Check sheet for the modelled part. Datum: model origin and axes. Units: mm. A direction names the side the tool comes from. Round coordinates to 2 decimals unless told otherwise and drop trailing zeros. Write each loop counter-clockwise with the first axis right and the second up, starting at its lowest first coordinate (ties: lowest second). Pieces come first, ordered by that corner, then holes. Notation, with made-up numbers: (39.25, -36.75) - (72.25, -36.75) arc R23 ccw to (72.25, -0.75) - close; hole circle Ø4 at (9.5, 79). An arc over 180 degrees is marked (long way). Use one line per item in the form item = value. Start each with the question number.
1) Section check D-D (y = 2.5). Record the boundary of the cut face in (x, z) (3 decimals), then the cut area to 3 significant figures.
2) Gauge pin test, flat ends, axial feed: P1, Ø5.5, axis at x = 85.852, z = -50.8, coming from the -Y side; P2, Ø1, axis at x = 86, y = 1.5, coming from the +Z side; P3, Ø1.6, axis at y = 1, z = -85.5, coming from the -X side. Record the tip position at first contact, or that the pin passes through.
3) Draft check along Z on faces 1 (the face through (44, 2, -101.065)), 2 (the face through (47.6, 1.61, -8.03)), 3 (the face through (34, 2, 0)). Enter one of: +Z half, -Z half, draft (parallel to the pull), parting line (faces both ways), or undercut.
4) Section check B-B (z = -82.55). Record the boundary of the cut face in (x, y) (3 decimals), then the cut area to 3 significant figures.
5) Section check A-A (x = 44.45). Record the boundary of the cut face in (y, z) (3 decimals).
6) Set-up check for faces 4 (the face through (88, 1.61, -53.14)), 5 (the face through (27.711, 2, -83)), 6 (the face through (68.072, 2, -19)), 7 (the face through (93.472, 2, -72)), 8 (the face through (64.9, 1.6, -103)): record each of +Z, -Z, +X, -X, +Y, -Y from which the full face is reachable in a straight line by a thin tool's end or side.
7) Section check C-C (z = -7.62). Record the boundary of the cut face in (x, y) (3 decimals), then the cut area to 3 significant figures.
8) Scan lines: probe 1 along X at (y, z) = (1, -7.5); probe 2 along Z at (x, y) = (79, 1.8); probe 3 along X at (y, z) = (0.9, -82.55). Record each from-to range of solid material in increasing order.
from build123d import *

# Parameters (mm, degrees)
SKETCH1_W           = 68.072
SKETCH1_H           = 38.1
SKETCH1_W_2         = 25.4
SKETCH1_H_2         = 68.072
BOSS_EXTRUDE1_DEPTH = 3.175
SKETCH2_R           = 3.175
CUT_EXTRUDE1_DEPTH  = 142.490596836
SKETCH3_W           = 34.0106
SKETCH3_H           = 54.542014323
BOSS_EXTRUDE2_DEPTH = 3.175


with BuildPart() as part:
    # Sketch1 → Boss-Extrude1 (new body)
    with BuildSketch(Plane(origin=(0, 0, 0), x_dir=(1, 0, 0), z_dir=(0, 1, 0))):
        with Locations((34.036, 19.05)):
            Rectangle(SKETCH1_W, SKETCH1_H)
        Polygon((68.072, 106.172), (68.072, 38.1), (0, 38.1), align=None)
        with Locations((80.772, 72.136)):
            Rectangle(SKETCH1_W_2, SKETCH1_H_2)
    extrude(amount=BOSS_EXTRUDE1_DEPTH)

    # Sketch2 → Cut-Extrude1 (cut, through all)
    with BuildSketch(Plane(origin=(0, 3.175, 0), x_dir=(1, 0, 0), z_dir=(0, 1, 0))):
        with Locations(Location((12.7, 7.62, 0), (0, 0, 270))):
            Circle(SKETCH2_R)
        with Locations(Location((44.45, 7.62, 0), (0, 0, 270))):
            Circle(SKETCH2_R)
        with Locations(Location((85.852, 50.8, 0), (0, 0, 270))):
            Circle(SKETCH2_R)
        with Locations(Location((85.852, 82.55, 0), (0, 0, 270))):
            Circle(SKETCH2_R)
    extrude(amount=-CUT_EXTRUDE1_DEPTH, mode=Mode.SUBTRACT)

    # Sketch3 → Boss-Extrude2 (add)
    with BuildSketch(Plane(origin=(0, 3.175, 0), x_dir=(1, 0, 0), z_dir=(0, 1, 0))):
        with Locations((44.7167, 73.793637407)):
            Rectangle(SKETCH3_W, SKETCH3_H)
    extrude(amount=-BOSS_EXTRUDE2_DEPTH)


solid = part.part
Results are:
q1.outline = (0, -38.1) - (27.711, -65.811) - (27.711, -101.065) - (61.722, -101.065) - (61.722, -99.822) - (68.072, -106.172) - (93.472, -106.172) - (93.472, -38.1) - (68.072, -38.1) - (68.072, 0) - (0, 0) - close; hole circle Ø6.35 at (12.7, -7.62); hole circle Ø6.35 at (44.45, -7.62); hole circle Ø6.35 at (85.852, -82.55); hole circle Ø6.35 at (85.852, -50.8)
q1.area = 7,130 mm²
q2.P1 = through
q2.P2 = -38.1
q2.P3 = 27.71
q3.face_1 = -Z half
q3.face_2 = undercut
q3.face_3 = +Z half
q4.outline = (27.711, 0) - (82.677, 0) - (82.677, 3.175) - (27.711, 3.175) - close; (89.027, 0) - (93.472, 0) - (93.472, 3.175) - (89.027, 3.175) - close
q4.area = 189 mm²
q5.outline = (0, -101.065) - (3.175, -101.065) - (3.175, -10.795) - (0, -10.795) - close; (0, -4.445) - (3.175, -4.445) - (3.175, 0) - (0, 0) - close
q6.face_4 = +Y, -Y
q6.face_5 = -Z, -X, +Y, -Y
q6.face_6 = +Z, +X, +Y, -Y
q6.face_7 = +Z, -Z, +X, +Y, -Y
q6.face_8 = -Z, +Y, -Y
q7.outline = (0, 0) - (9.525, 0) - (9.525, 3.175) - (0, 3.175) - close; (15.875, 0) - (41.275, 0) - (41.275, 3.175) - (15.875, 3.175) - close; (47.625, 0) - (68.072, 0) - (68.072, 3.175) - (47.625, 3.175) - close
q7.area = 176 mm²
q8.probe_1 = 0 to 9.53, 15.87 to 41.28, 47.62 to 68.07
q8.probe_2 = -106.17 to -38.1
q8.probe_3 = 27.71 to 82.68, 89.03 to 93.47
